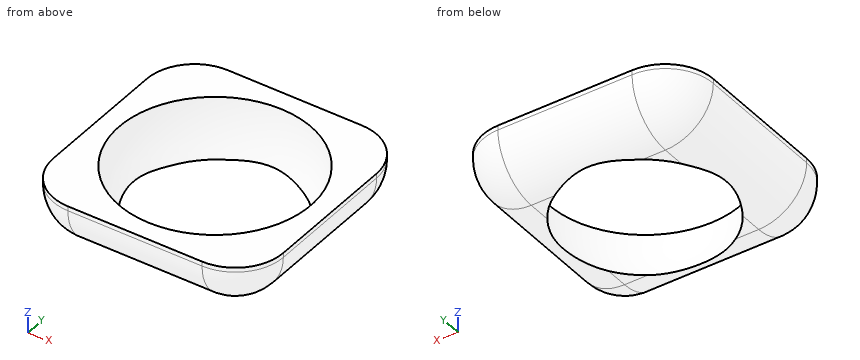
from build123d import *

# Parameters (mm, degrees)
SKETCH2_W           = 24
SKETCH2_H           = 24
BOSS_EXTRUDE1_DEPTH = 10.5
CUT_EXTRUDE1_DEPTH  = 36.528157847
FILLET1_R           = 5


with BuildPart() as part:
    # Sketch2 → Boss-Extrude1 (new body)
    with BuildSketch(Plane.XY):
        with Locations((12, 12)):
            Rectangle(SKETCH2_W, SKETCH2_H)
    extrude(amount=BOSS_EXTRUDE1_DEPTH)

    # Sketch4 → Cut-Revolve1 (revolve, cut)
    with BuildSketch(Plane.XY.offset(10.5)):
        with BuildLine():
            Line((12, 22), (12, 2))
            ThreePointArc((12, 2), (2, 12), (12, 22))
        make_face()
    revolve(axis=Axis((12, 22, 10.5), (0, -1, 0)), mode=Mode.SUBTRACT)

    # Sketch6 → Cut-Extrude1 (cut, through all)
    with BuildSketch(Plane(origin=(24, 0, 0), x_dir=(0, 0, -1), z_dir=(1, 0, 0))):
        Polygon((0, 24), (-3.026616613, 24), (-5.026616613, 24), (-5.026616613, 0), (-3.026616613, 0), (0, 0), align=None)
    extrude(amount=-CUT_EXTRUDE1_DEPTH, mode=Mode.SUBTRACT)

    # Fillet1
    # the kernel refuses this fillet: 5 mm, written as the material it takes off along each edge
    with BuildSketch(Plane(origin=(5, 19, 10.026616613), x_dir=(-1, 0, 0), z_dir=(0, 0, -1))) as fillet1_piece_1_section:
        Polygon((0, 0), (FILLET1_R, 0), (FILLET1_R, FILLET1_R), (0, FILLET1_R), align=None)
    fillet1_piece_1 = extrude(amount=FILLET1_R, mode=Mode.PRIVATE)
    fillet1_piece_1 = fillet1_piece_1 - Plane(origin=(5, 19, 10.026616613), x_dir=(0.7071067811865475, -0.7071067811865475, 0), z_dir=(0, 0, -1)) * Sphere(FILLET1_R, mode=Mode.PRIVATE)
    add(fillet1_piece_1, mode=Mode.SUBTRACT)
    with BuildSketch(Plane(origin=(5, 5, 10.026616613), x_dir=(0, 0, -1), z_dir=(0, -1, 0))) as fillet1_piece_2_section:
        Polygon((0, 0), (FILLET1_R, 0), (FILLET1_R, -FILLET1_R), (0, -FILLET1_R), align=None)
    fillet1_piece_2 = extrude(amount=FILLET1_R, mode=Mode.PRIVATE)
    fillet1_piece_2 = fillet1_piece_2 - Plane(origin=(5, 5, 10.026616613), x_dir=(0.7071067811865475, 0, 0.7071067811865475), z_dir=(0, -1, 0)) * Sphere(FILLET1_R, mode=Mode.PRIVATE)
    add(fillet1_piece_2, mode=Mode.SUBTRACT)
    with BuildSketch(Plane(origin=(19, 5, 10.026616613), x_dir=(0, 0, -1), z_dir=(0, -1, 0))) as fillet1_piece_3_section:
        Polygon((0, 0), (FILLET1_R, 0), (FILLET1_R, FILLET1_R), (0, FILLET1_R), align=None)
    fillet1_piece_3 = extrude(amount=FILLET1_R, mode=Mode.PRIVATE)
    fillet1_piece_3 = fillet1_piece_3 - Plane(origin=(19, 5, 10.026616613), x_dir=(-0.7071067811865475, 0, 0.7071067811865475), z_dir=(0, -1, 0)) * Sphere(FILLET1_R, mode=Mode.PRIVATE)
    add(fillet1_piece_3, mode=Mode.SUBTRACT)
    with BuildSketch(Plane(origin=(19, 19, 10.026616613), x_dir=(1, 0, 0), z_dir=(0, 0, -1))) as fillet1_piece_4_section:
        Polygon((0, 0), (FILLET1_R, 0), (FILLET1_R, -FILLET1_R), (0, -FILLET1_R), align=None)
    fillet1_piece_4 = extrude(amount=FILLET1_R, mode=Mode.PRIVATE)
    fillet1_piece_4 = fillet1_piece_4 - Plane(origin=(19, 19, 10.026616613), x_dir=(-0.7071067811865475, -0.7071067811865475, 0), z_dir=(0, 0, -1)) * Sphere(FILLET1_R, mode=Mode.PRIVATE)
    add(fillet1_piece_4, mode=Mode.SUBTRACT)
    with BuildSketch(Plane(origin=(0, 19, 5.026616613), x_dir=(1, 0, 0), z_dir=(0, -1, 0)), Plane(origin=(19, 0, 5.026616613), x_dir=(0, 0, 1), z_dir=(-1, 0, 0)), Plane(origin=(19, 24, 5.026616613), x_dir=(0, -1, 0), z_dir=(-1, 0, 0))) as fillet1_piece_5:
        with BuildLine():
            CenterArc((FILLET1_R, FILLET1_R), FILLET1_R, 180, 90)
            Line((0, FILLET1_R), (0, 0))
            Line((0, 0), (FILLET1_R, 0))
        make_face()
    extrude(amount=14, mode=Mode.SUBTRACT)
    with BuildSketch(Plane(origin=(24, 19, 5.026616613), x_dir=(-1, 0, 0), z_dir=(0, -1, 0))) as fillet1_piece_6:
        with BuildLine():
            CenterArc((FILLET1_R, -FILLET1_R), FILLET1_R, 90, 90)
            Line((0, -FILLET1_R), (0, 0))
            Line((0, 0), (FILLET1_R, 0))
        make_face()
    extrude(amount=14, mode=Mode.SUBTRACT)
    with BuildSketch(Plane(origin=(0, 24, 10.026616613), x_dir=(0, -1, 0), z_dir=(0, 0, 1)), Plane(origin=(0, 0, 10.026616613), x_dir=(1, 0, 0), z_dir=(0, 0, 1))) as fillet1_piece_7:
        with BuildLine():
            CenterArc((FILLET1_R, FILLET1_R), FILLET1_R, 180, 90)
            Line((0, FILLET1_R), (0, 0))
            Line((0, 0), (FILLET1_R, 0))
        make_face()
    extrude(amount=12.973383387, mode=Mode.SUBTRACT)
    with BuildSketch(Plane(origin=(24, 24, 10.026616613), x_dir=(0, -1, 0), z_dir=(0, 0, 1)), Plane(origin=(24, 0, 10.026616613), x_dir=(-1, 0, 0), z_dir=(0, 0, 1))) as fillet1_piece_8:
        with BuildLine():
            CenterArc((FILLET1_R, -FILLET1_R), FILLET1_R, 90, 90)
            Line((0, -FILLET1_R), (0, 0))
            Line((0, 0), (FILLET1_R, 0))
        make_face()
    extrude(amount=12.973383387, mode=Mode.SUBTRACT)


solid = part.part
Work out the finished part from the listing and answer in its coordinate system (mm). Round coordinates to 2 decimals unless told otherwise and drop trailing zeros. Write each loop counter-clockwise with the first axis right and the second up, starting at its lowest first coordinate (ties: lowest second). Pieces come first, ordered by that corner, then holes.
1) A cutting plane is placed at C-C (y = 10.25). Give the vertices of the cut face in (x, z), plus the area to 3 significant figures.
2) A cutting plane is placed at A-A (x = 15.25). Give the vertices of the cut face in (y, z).
3) A cutting plane is placed at B-B (z = 9). Give the vertices of the cut face in (x, y).
4) Straight lines are drawn through the part: line 1 (Y direction, x = 15.25, z = 9.7); line 2 (X direction, y = 7.75, z = 5.6); line 3 (X direction, y = 20.75, z = 7.6). For each, find the intervals that lie inside material, in ascending order.
5) A cutting plane is placed at D-D (x = 1.5). Give the vertices of the cut face in (y, z).
Completed:
1. outline: (0, 10.03) arc R5 ccw to (3.7, 5.2) arc R9.85 cw to (2.15, 10.5) - (0, 10.5) - close; (20.3, 5.2) arc R5 ccw to (24, 10.03) - (24, 10.5) - (21.85, 10.5) arc R9.85 cw to start
1. area: 18.8 mm2
2. outline: (0, 10.03) arc R5 ccw to (4.25, 5.08) arc R9.46 cw to (2.54, 10.5) - (0, 10.5) - close; (19.75, 5.08) arc R5 ccw to (24, 10.03) - (24, 10.5) - (21.46, 10.5) arc R9.46 cw to start
3. outline: (0.11, 5) arc R4.89 ccw to (5, 0.11) - (19, 0.11) arc R4.89 ccw to (23.89, 5) - (23.89, 19) arc R4.89 ccw to (19, 23.89) - (5, 23.89) arc R4.89 ccw to (0.11, 19) - close; hole circle Ø19.77 at (12, 12)
4. line 1: y = 0.01 to 2.58, 21.42 to 23.99
4. line 2: x = 2.68 to 4.39, 19.61 to 21.32
4. line 3: x = 0.99 to 8.12, 15.88 to 23.01
5. outline: (1.43, 10.03) arc R3.57 ccw to (5, 6.46) - (19, 6.46) arc R3.57 ccw to (22.57, 10.03) - (22.57, 10.5) - (1.43, 10.5) - close
